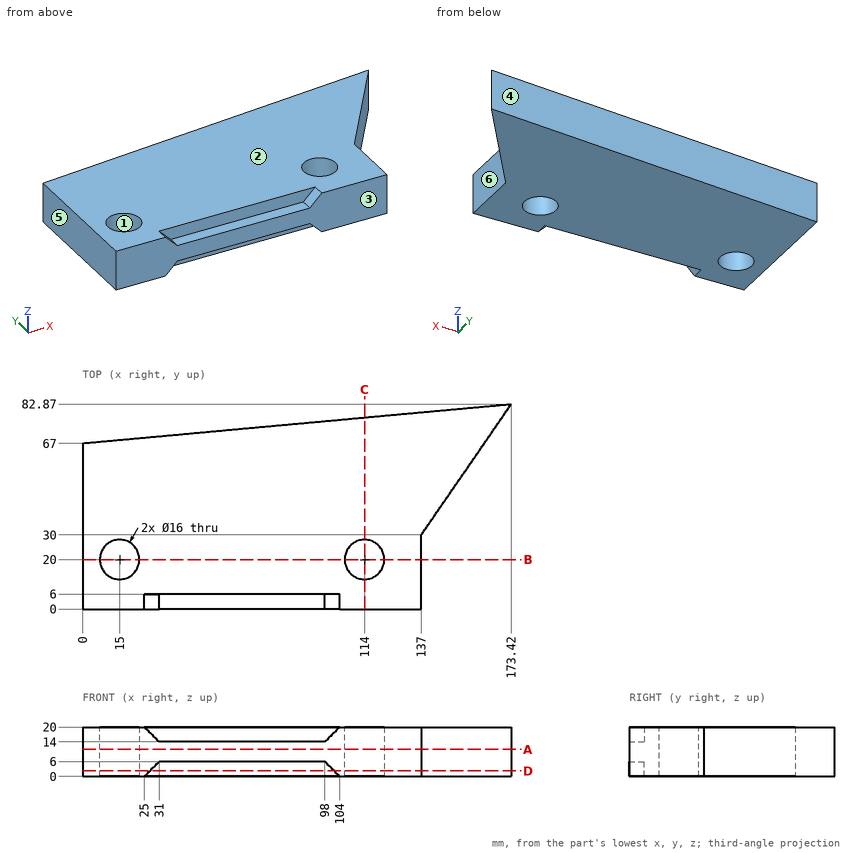
Part print with two shaded views. Sizes in mm from the minimum x, y, z corner. A direction names the side the tool comes from. Coordinates: 2 decimals unless noted, no trailing zeros. Order: outer loops, then holes, each group sorted by start corner. A loop starts at its lowest first (then second) coordinate and runs counter-clockwise, first axis right, second up.
(1) Mould opens along Y. For the marked faces 1, 2, 3 and 4 say: released by +Y, released by -Y, zero draft, split by the parting line, or undercut.
Solution:
face 1: undercut
face 2: zero draft
face 3: released by -Y
face 4: released by +Y
(2) Saw through at D-D, the plane z = 2.25. Write the cut outline in (x, y).
Solution:
outline: (0, 0) - (27.25, 0) - (27.25, 6) - (101.75, 6) - (101.75, 0) - (137, 0) - (137, 30) - (173.42, 82.87) - (0, 67) - close; hole circle Ø16 at (15, 20); hole circle Ø16 at (114, 20)
(3) Saw through at B-B, the plane y = 20. Write the cut outline in (x, z), and give its area (3 significant figures).
Solution:
outline: (0, 0) - (7, 0) - (7, 20) - (0, 20) - close; (23, 0) - (106, 0) - (106, 20) - (23, 20) - close; (122, 0) - (137, 0) - (137, 20) - (122, 20) - close
area: 2,100 mm2
(4) Which spindle directions (+Z, -Z, +X, -X, +Y, -Y) get a long thin tool onto all of the face, cutting with end or side? Do the marked faces 5 and 6. Say none if no direction does.
Solution:
face 5: +Z, -Z, -X, +Y, -Y
face 6: +Z, -Z, +X, -Y
(5) Saw through at A-A, the plane z = 11. Write the cut outline in (x, y).
Solution:
outline: (0, 0) - (137, 0) - (137, 30) - (173.42, 82.87) - (0, 67) - close; hole circle Ø16 at (15, 20); hole circle Ø16 at (114, 20)
(6) Saw through at C-C, the plane x = 114. Write the cut outline in (y, z), and give its area (3 significant figures).
Solution:
outline: (0, 0) - (12, 0) - (12, 20) - (0, 20) - close; (28, 0) - (77.43, 0) - (77.43, 20) - (28, 20) - close
area: 1,230 mm2
(7) Pin check, flat tips, straight feed: pin 1 Ø4 at (x, z) = (75.5, 7) entering from +Y; pin 2 Ø6.5 at (x, y) = (64, 1.5) entering from +Z; pin 3 Ø4 at (y, z) = (30, 14) entering from +X. Stop position of each tip, or through.
Solution:
pin 1: stops at y = 74.09
pin 2: stops at z = 14
pin 3: stops at x = 138.38
(8) Drill centre lines: L1, parallel to X at y = 24.5, z = 9; L2, parallel to X at y = 22, z = 17.5; L3, parallel to Y at x = 114.5, z = 2. Where is each one in solid material? Low to high.
Solution:
L1: x = 0 to 8.39, 21.61 to 107.39, 120.61 to 137
L2: x = 0 to 7.25, 22.75 to 106.25, 121.75 to 137
L3: y = 0 to 12.02, 27.98 to 77.48
